CAD build for the part. Positions are in the model's coordinates, mm. A direction names the side the tool comes from. Coordinates: 2 decimals unless noted, no trailing zeros. Write each loop counter-clockwise with the first axis right and the second up, starting at its lowest first coordinate (ties: lowest second). Pieces come first, ordered by that corner, then holes. Notation, with made-up numbers: (33, -31) - (76, -31) arc R20 cw to (76, -7) - close; hole circle Ø3 at (67, 89.5). An arc over 180 degrees is marked (long way). One line per question, with ' | ' between items. Start each with the question number.
1. Band-saw the part on A-A, the plane z = 0. Write the cut outline in (x, y) (3 decimals), then the cut area to 3 significant figures.
2. Flat gauge pins, fed straight in: P1, Ø10, axis at x = -71, z = -35, coming from the +Y side; P2, Ø22, axis at x = 0, z = 0, coming from the -Y side; P3, Ø1.5, axis at y = -56.5, z = -27, coming from the -X side; P4, Ø6, axis at x = 24.5, y = -7.5, coming from the +Z side. Where does each tip first touch, or does it go through?
3. Which spindle directions (+Z, -Z, +X, -X, +Y, -Y) get a long thin tool onto all of the face, cutting with end or side? Do faces 1 (the cylindrical face through (-60.278, -79.249, 0.423)), 2 (the flat face through (19, -78.476, -1)). Say none if no direction does.
4. Two-plate mould, pull along X, no slides. Class faces 3 (the cylindrical face through (93.233, -16.101, 20.703)), 4 (the cylindrical face through (57.185, -13.607, 74.579)), 5 (the flat face through (63, 47, 70)): +X half, -X half, draft (parallel to the pull), parting line (faces both ways), or undercut.
5. Probe line 1 (X direction, y = -79, z = 0) (3 decimals); line 2 (Y direction, x = 17, z = -13.5); line 3 (X direction, y = -40.5, z = 0). List the from-to ranges inside material, lowest first.
6. Band-saw the part on C-C, the plane y = 25. Write the cut outline in (x, z), then the cut area to 3 significant figures.
7. Band-saw the part on B-B, the plane x = 0. Write the cut outline in (y, z) (3 decimals).
from build123d import *

# Parameters (mm, degrees)
CUT_EXTRUDE2_REACH = 187.394
MOTOR_HOLE_R       = 18.415
MOTOR_HOLE_R_2     = 3.25
FILLET1_R          = 2.54


with BuildPart() as part:
    # Compartment → Revolve1 (revolve)
    with BuildSketch(Plane.XY, mode=Mode.PRIVATE) as revolve1_sk:
        Polygon((95.504, -80), (0, -80), (0, -78.476), (93.98, -78.476), (93.98, 47), (95.504, 47), align=None)
    revolve(revolve1_sk.sketch.rotate(Axis((0, 0, 0), (0, 1, 0)), 90), axis=Axis((0, 0, 0), (0, 1, 0)))

    # Motor Hole → Cut-Extrude2 (cut, up to next)
    with BuildSketch(Plane.XZ.offset(80), mode=Mode.PRIVATE) as cut_extrude2_sk1:
        with Locations(Location((0, 0, 0), (0, 0, 270))):
            Circle(MOTOR_HOLE_R)
    cut_extrude2_tool1 = extrude(cut_extrude2_sk1.sketch, amount=-CUT_EXTRUDE2_REACH, mode=Mode.PRIVATE) & part.part
    # Motor Hole → Cut-Extrude2 (cut, up to next)
    with BuildSketch(Plane.XZ.offset(80), mode=Mode.PRIVATE) as cut_extrude2_sk2:
        with Locations(Location((0, 63.5, 0), (0, 0, 270))):
            Circle(MOTOR_HOLE_R_2)
    cut_extrude2_tool2 = extrude(cut_extrude2_sk2.sketch, amount=-CUT_EXTRUDE2_REACH, mode=Mode.PRIVATE) & part.part
    # Motor Hole → Cut-Extrude2 (cut, up to next)
    with BuildSketch(Plane.XZ.offset(80), mode=Mode.PRIVATE) as cut_extrude2_sk3:
        with Locations(Location((63.5, 0, 0), (0, 0, 270))):
            Circle(MOTOR_HOLE_R_2)
    cut_extrude2_tool3 = extrude(cut_extrude2_sk3.sketch, amount=-CUT_EXTRUDE2_REACH, mode=Mode.PRIVATE) & part.part
    # Motor Hole → Cut-Extrude2 (cut, up to next)
    with BuildSketch(Plane.XZ.offset(80), mode=Mode.PRIVATE) as cut_extrude2_sk4:
        with Locations(Location((0, -63.5, 0), (0, 0, 270))):
            Circle(MOTOR_HOLE_R_2)
    cut_extrude2_tool4 = extrude(cut_extrude2_sk4.sketch, amount=-CUT_EXTRUDE2_REACH, mode=Mode.PRIVATE) & part.part
    # Motor Hole → Cut-Extrude2 (cut, up to next)
    with BuildSketch(Plane.XZ.offset(80), mode=Mode.PRIVATE) as cut_extrude2_sk5:
        with Locations(Location((-63.5, 0, 0), (0, 0, 270))):
            Circle(MOTOR_HOLE_R_2)
    cut_extrude2_tool5 = extrude(cut_extrude2_sk5.sketch, amount=-CUT_EXTRUDE2_REACH, mode=Mode.PRIVATE) & part.part
    add(cut_extrude2_tool1.solids().sort_by_distance((0, -80, 0))[0], mode=Mode.SUBTRACT)
    add(cut_extrude2_tool2.solids().sort_by_distance((0, -80, 63.5))[0], mode=Mode.SUBTRACT)
    add(cut_extrude2_tool3.solids().sort_by_distance((63.5, -80, 0))[0], mode=Mode.SUBTRACT)
    add(cut_extrude2_tool4.solids().sort_by_distance((0, -80, -63.5))[0], mode=Mode.SUBTRACT)
    add(cut_extrude2_tool5.solids().sort_by_distance((-63.5, -80, 0))[0], mode=Mode.SUBTRACT)

    # Fillet1
    fillet1_edges = [part.edges().sort_by_distance(p)[0] for p in [
        (0, -78.476, 93.98),
        (0, -80, 95.504),
    ]]
    fillet(fillet1_edges, radius=FILLET1_R)


solid = part.part
Filled in:
1) outline: (-95.504, -77.46) arc R2.54 ccw to (-92.964, -80) - (-66.75, -80) - (-66.75, -78.476) - (-91.44, -78.476) arc R2.54 cw to (-93.98, -75.936) - (-93.98, 47) - (-95.504, 47) - close; (-60.25, -80) - (-18.415, -80) - (-18.415, -78.476) - (-60.25, -78.476) - close; (18.415, -80) - (60.25, -80) - (60.25, -78.476) - (18.415, -78.476) - close; (66.75, -80) - (92.964, -80) arc R2.54 ccw to (95.504, -77.46) - (95.504, 47) - (93.98, 47) - (93.98, -75.936) arc R2.54 cw to (91.44, -78.476) - (66.75, -78.476) - close | area: 598 mm²
2) P1: stops at y = -78.48 | P2: passes through | P3: stops at x = -91.83 | P4: stops at z = 93.05
3) face 1: +Y, -Y | face 2: +Y
4) face 3: parting line | face 4: undercut | face 5: draft
5) line 1: x = -94.984 to -66.75, -60.25 to -18.415, 18.415 to 60.25, 66.75 to 94.984 | line 2: y = -80 to -78.48 | line 3: x = -95.5 to -93.98, 93.98 to 95.5
6) outline: circle Ø191.01 at (0, 0); hole circle Ø187.96 at (0, 0) | area: 907 mm²
7) outline: (-80, -92.964) arc R2.54 ccw to (-77.46, -95.504) - (47, -95.504) - (47, -93.98) - (-75.936, -93.98) arc R2.54 cw to (-78.476, -91.44) - (-78.476, -66.75) - (-80, -66.75) - close; (-80, -60.25) - (-78.476, -60.25) - (-78.476, -18.415) - (-80, -18.415) - close; (-80, 18.415) - (-78.476, 18.415) - (-78.476, 60.25) - (-80, 60.25) - close; (-80, 66.75) - (-78.476, 66.75) - (-78.476, 91.44) arc R2.54 cw to (-75.936, 93.98) - (47, 93.98) - (47, 95.504) - (-77.46, 95.504) arc R2.54 ccw to (-80, 92.964) - close
